Study the drawing (mm; zero at the part's minimum x, y, z) and answer. A direction names the side the tool comes from. Give positions to 0.01 mm unless a question says otherwise; leave off trailing zeros. Write each loop counter-clockwise with the first axis right and the second up, starting at its lowest first coordinate (ties: lowest second). Pieces come first, ordered by that corner, then holes. Notation, with made-up numbers: M 87.25,7 L 110.25,7 A30 cw 110.25,45 Z; hole C -16,48 d10. An arc over 180 degrees is marked long. Use a Markdown table: item, result. Add a question column.
Item 1: A cutting plane is placed at C-C on x = 171.5. Determine the outline of the cut face in (y, z).
Item 2: A cutting plane is placed at D-D on y = 65. Determine the outline of the cut face in (x, z).
Item 3: Consider probe 1 along X at (y, z) = (157.8, 14.5) (1 decimal); probe 2 along X at (y, z) = (57, 35.5); probe 3 along Z at (x, y) = (41, 64.5). Determine where each line is inside the solid, lowest interval first. Write a range as [from, to].
Item 4: For the marked faces 1, 2 and 3, determine the directions among +Z, -Z, +X, -X, +Y, -Y from which every point of the face is accessible in a straight line to the end or side of a thin tool.
Item 5: Given P1, Ø4, axis at x = 106.36, y = 157.8, coming from the -Z side; P2, Ø19, axis at x = 19, y = 109, coming from the +Z side; P3, Ø1.5, axis at y = 108, z = 38.5, coming from the -X side; P4, Ø2, axis at y = 55, z = 21.5, coming from the -X side, each flat-ended and moving along its own axis, determine where each tip first touches the part or whether it passes through.
Item 6: A cutting plane is placed at B-B on y = 101. Determine the outline of the cut face in (x, z).
Item 7: A cutting plane is placed at A-A on z = 44. Determine the outline of the cut face in (x, y).
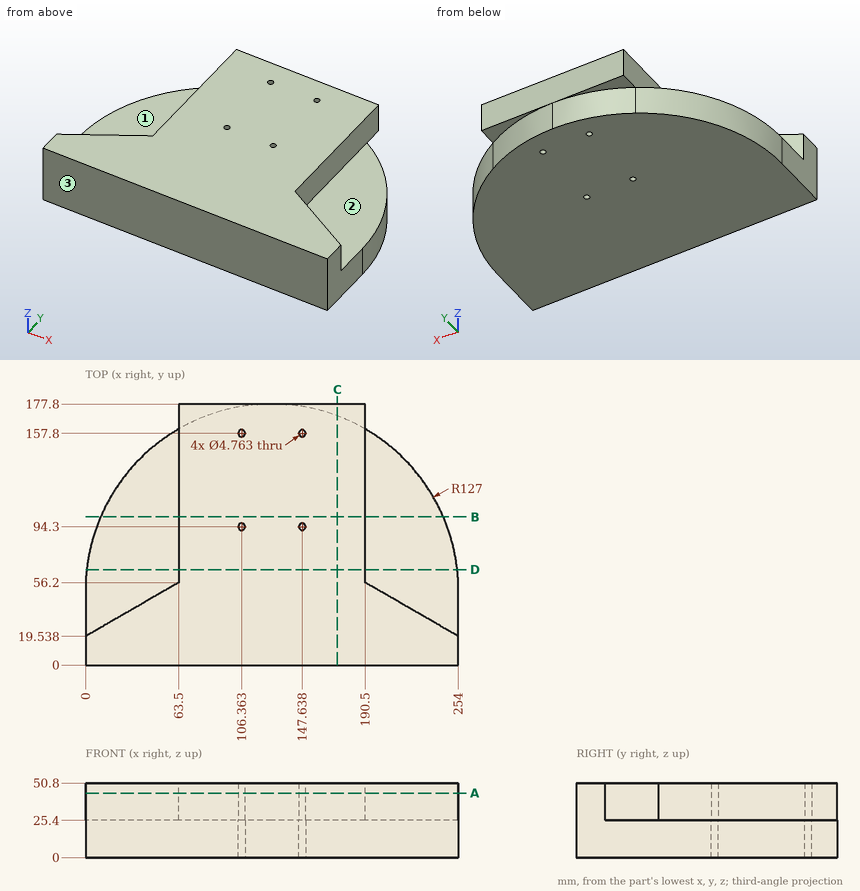
Filled in:
| question | item | result |
|---|---|---|
| 1 | outline | M 0,0 L 169.75,0 L 169.75,25.4 L 177.8,25.4 L 177.8,50.8 L 0,50.8 Z |
| 2 | outline | M 0.8,0 L 253.2,0 L 253.2,25.4 L 190.5,25.4 L 190.5,50.8 L 63.5,50.8 L 63.5,25.4 L 0.8,25.4 Z |
| 3 | probe 1 | [58.6, 104], [108.7, 145.3], [150, 195.4] |
| 3 | probe 2 | [63.5, 190.5] |
| 3 | probe 3 | [0, 25.4] |
| 4 | face 1 | +Z, -X, +Y |
| 4 | face 2 | +Z, +X, +Y |
| 4 | face 3 | +Z, -Z, +X, -X, -Y |
| 5 | P1 | through |
| 5 | P2 | z = 25.4 |
| 5 | P3 | x = 63.5 |
| 5 | P4 | x = 0.04 |
| 6 | outline | M 10.34,0 L 243.66,0 L 243.66,25.4 L 190.5,25.4 L 190.5,50.8 L 63.5,50.8 L 63.5,25.4 L 10.34,25.4 Z |
| 7 | outline | M 0,0 L 254,0 L 254,19.54 L 190.5,56.2 L 190.5,177.8 L 63.5,177.8 L 63.5,56.2 L 0,19.54 Z; hole C 106.36,94.3 d4.76; hole C 106.36,157.8 d4.76; hole C 147.64,94.3 d4.76; hole C 147.64,157.8 d4.76 |
